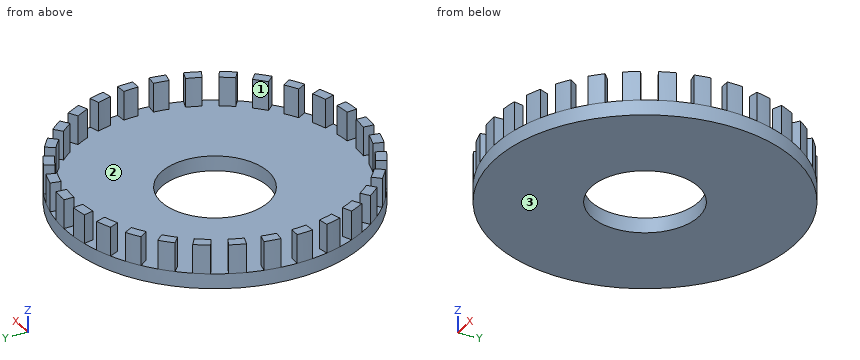
from build123d import *

# Parameters (mm, degrees)
SKETCH1_R           = 30
SKETCH1_R_2         = 10.715625
BOSS_EXTRUDE1_DEPTH = 3
BOSS_EXTRUDE2_DEPTH = 5.8
CIRPATTERN1_COUNT   = 30


with BuildPart() as part:
    # Sketch1 → Boss-Extrude1 (new body)
    with BuildSketch(Plane.XY):
        Circle(SKETCH1_R)
        Circle(SKETCH1_R_2, mode=Mode.SUBTRACT)
    extrude(amount=BOSS_EXTRUDE1_DEPTH)

    # Sketch2 → Boss-Extrude2 (add)
    with BuildSketch(Plane.XY.offset(3)):
        with BuildLine():
            Line((0, 30), (0, 28))
            ThreePointArc((0, 28), (1.465406775, 27.961626973), (2.926796971, 27.84661307))
            Line((2.926796971, 27.84661307), (3.135853898, 29.835656861))
            ThreePointArc((3.135853898, 29.835656861), (1.570078687, 29.958886043), (0, 30))
        make_face()
    boss_extrude2 = extrude(amount=BOSS_EXTRUDE2_DEPTH)

    # CirPattern1: Boss-Extrude2 ×30 about axis
    cirpattern1_axis = Axis((0, 0, 0), (0, 0, 1))
    for i in range(1, CIRPATTERN1_COUNT):
        add(boss_extrude2.rotate(cirpattern1_axis, i * 360 / CIRPATTERN1_COUNT))


solid = part.part
Verification items for the finished model (mm, model axes). Face numbers are marked on the shaded views. Coordinates: 2 decimals unless noted, no trailing zeros. Write each loop counter-clockwise with the first axis right and the second up, starting at its lowest first coordinate (ties: lowest second). Pieces come first, ordered by that corner, then holes. Notation, with made-up numbers: M 1,31.25 L 29,31.25 A13 cw 29,54.25 Z; hole C 45,32 d10. An arc over 180 degrees is marked long. Use a Markdown table: item, result.
Q1. Draft check along Y on the marked faces 1, 2 and 3. Enter one of: +Y half, -Y half, draft (parallel to the pull), parting line (faces both ways), or undercut.
Reply:
| item | result |
|---|---|
| face 1 | undercut |
| face 2 | undercut |
| face 3 | draft |
Q2. Sectioned sample at B-B, the plane x = 1. Record the boundary of the cut face in (y, z).
Reply:
| item | result |
|---|---|
| outline | M -29.98,0 L -10.67,0 L -10.67,3 L -29.98,3 Z; M 10.67,0 L 29.98,0 L 29.98,8.8 L 27.98,8.8 L 27.98,3 L 10.67,3 Z |
Q3. Go/stop test with flat-tipped pins: P1, Ø2, axis at y = 15.5, z = 7.5, coming from the +X side; P2, Ø18, axis at x = -13, y = -7, coming from the +Z side; P3, Ø2, axis at x = 9, z = 2.5, coming from the -Y side; P4, Ø1, axis at x = -9, y = -2, coming from the -Z side. Record where each tip stops, or that it passes through.
Reply:
| item | result |
|---|---|
| P1 | stops at x = 26.26 |
| P2 | stops at z = 3 |
| P3 | stops at y = -28.91 |
| P4 | passes through |
Q4. Sectioned sample at A-A, the plane z = 7. Count the separate pieces of the cut face and the enclosed holes in it, plus the area to 3 significant figures.
Reply:
| item | result |
|---|---|
| separate pieces | 30 |
| enclosed holes | 0 |
| area | 182 mm² |
Q5. Thickness scan on line 1 (Y direction, x = 0, z = 1.9); line 2 (X direction, y = -12, z = 6.25); line 3 (Z direction, x = -4, y = 20.5). Record the ranges inside material, lowest first.
Reply:
| item | result |
|---|---|
| line 1 | y = -30 to -10.72, 10.72 to 30 |
| line 2 | x = -26.95 to -25.3, 26.95 to 27.5 |
| line 3 | z = 0 to 3 |
